from build123d import *

# Parameters (mm, degrees)
SKETCH1_W           = 5
SKETCH1_H           = 50
BOSS_EXTRUDE1_DEPTH = 5
SKETCH2_W           = 10
SKETCH2_H           = 5
BOSS_EXTRUDE2_DEPTH = 10
SKETCH3_R           = 1
CUT_EXTRUDE1_DEPTH  = 47.97073557


with BuildPart() as part:
    # Sketch1 → Boss-Extrude1 (new, symmetric)
    with BuildSketch(Plane.XY):
        Rectangle(SKETCH1_W, SKETCH1_H)
    extrude(amount=BOSS_EXTRUDE1_DEPTH, both=True)

    # Sketch2 → Boss-Extrude2 (add)
    with BuildSketch(Plane.ZY.offset(2.5)):
        with Locations((0, -22.5)):
            Rectangle(SKETCH2_W, SKETCH2_H)
    extrude(amount=BOSS_EXTRUDE2_DEPTH)

    # Sketch3 → Cut-Extrude1 (cut, through all)
    with BuildSketch(Plane(origin=(0, -20, 0), x_dir=(1, 0, 0), z_dir=(0, 1, 0))):
        with Locations(Location((-7.5, 2.5, 0), (0, 0, 270))):
            Circle(SKETCH3_R)
        with Locations(Location((-7.5, -2.5, 0), (0, 0, 270))):
            Circle(SKETCH3_R)
    extrude(amount=-CUT_EXTRUDE1_DEPTH, mode=Mode.SUBTRACT)


solid = part.part
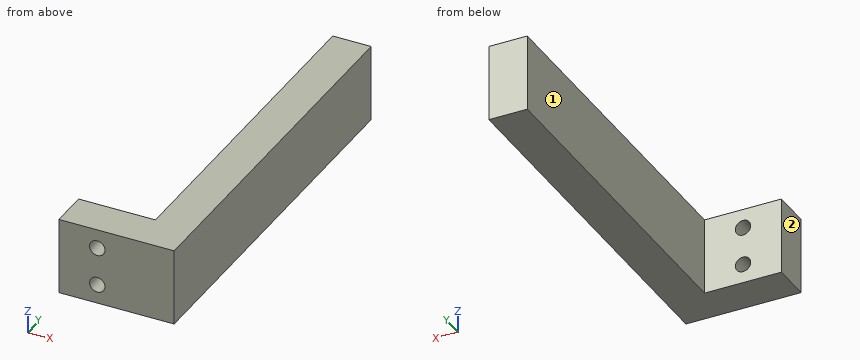
Here's how the part is built. I have some questions about the finished solid (model axes, mm). Face numbers are marked on the shaded views. A direction names the side the tool comes from. Give positions to 0.01 mm unless a question says otherwise; leave off trailing zeros. Order: outer loops, then holes, each group sorted by start corner. A loop starts at its lowest first (then second) coordinate and runs counter-clockwise, first axis right, second up. Notation, with made-up numbers: (32.25, 75) -> (73.25, 75) arc R29 ccw to (73.25, 103) -> close; hole circle Ø4 at (53, 87.25). An arc over 180 degrees is marked (long way). One line per item, written item: value. Start each with the question number.
1. Imagine slicing it at A-A, the plane z = -2.5. List the corners of the cut face in (x, y) for me.
2. Imagine slicing it at C-C, the plane y = 8. List the corners of the cut face in (x, z) for me, plus the area to 3 significant figures.
3. Imagine slicing it at B-B, the plane x = -7.5. List the corners of the cut face in (y, z) for me, plus the area to 3 significant figures.
4. I need wall thicknesses on probe 1 along X at (y, z) = (-22.65, -2.5); probe 2 along X at (y, z) = (17, -3.5); probe 3 along Y at (x, z) = (-10.25, -3.75). Which ranges of each line are inside material? Lowest first, please. Write a range as from..to.
5. For the marked faces 1 and 2, which set-ups out of +Z, -Z, +X, -X, +Y, -Y let a thin tool reach every point of the face, with its end or its side?
6. Will these pins go through, and if not, where does the flat tip stop? pin 1 Ø5 at (x, z) = (-8, 2.5) entering from +Y; pin 2 Ø6 at (y, z) = (15, -3.5) entering from -X.
Values follow:
1. outline: (-12.5, -25) -> (-8.5, -25) -> (-8.5, -20) -> (-12.5, -20) -> close; (-6.5, -25) -> (2.5, -25) -> (2.5, 25) -> (-2.5, 25) -> (-2.5, -20) -> (-6.5, -20) -> close
2. outline: (-2.5, -5) -> (2.5, -5) -> (2.5, 5) -> (-2.5, 5) -> close
2. area: 50.0 mm2
3. outline: (-25, -5) -> (-20, -5) -> (-20, -3.5) -> (-25, -3.5) -> close; (-25, -1.5) -> (-20, -1.5) -> (-20, 1.5) -> (-25, 1.5) -> close; (-25, 3.5) -> (-20, 3.5) -> (-20, 5) -> (-25, 5) -> close
3. area: 30.0 mm2
4. probe 1: x = -12.5..-8.5, -6.5..2.5
4. probe 2: x = -2.5..2.5
4. probe 3: y = -25..-20
5. face 1: +Z, -Z, -X, +Y
5. face 2: +Z, -Z, -X, +Y, -Y
6. pin 1: stops at y = -20
6. pin 2: stops at x = -2.5
